Read the model definition and answer for the solid it produces. Units are mm, in the model's axes. Coordinates: 2 decimals unless noted, no trailing zeros. Write each loop counter-clockwise with the first axis right and the second up, starting at its lowest first coordinate (ties: lowest second). Pieces come first, ordered by that corner, then holes.
Item 1: Straight lines are drawn through the part: probe 1 along Z at (x, y) = (-29.75, 6.15); probe 2 along X at (y, z) = (7.3, -115); probe 3 along Z at (x, y) = (-59, 5.95). For each, find the intervals that lie inside material, in ascending order.
Item 2: Each of these flat-tipped pins is pushed along its axis until it touches: P1, Ø1.4, axis at x = -59.75, z = -108, coming from the -Y side; P2, Ø3, axis at x = -29.75, z = -115, coming from the +Y side. Where does it stop, or does it pass through?
Item 3: Section A-A (z = -115) is taken. Give the vertices of the cut face in (x, y), then the cut area to 3 significant figures.
Item 4: Section B-B (x = -59.75) is taken. Give the vertices of the cut face in (y, z).
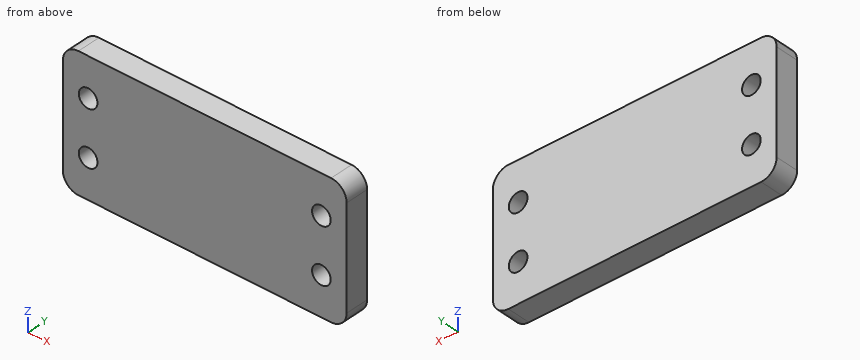
from build123d import *

# Parameters (mm, degrees)
CYLINDER015_R     = 1.2
CYLINDER015_DEPTH = 10
CYLINDER016_R     = 1.2
CYLINDER016_DEPTH = 10
CYLINDER012_R     = 1.2
CYLINDER012_DEPTH = 10
CYLINDER014_R     = 1.2
CYLINDER014_DEPTH = 10
BOX007_W          = 36.5
BOX007_H          = 3
BOX007_DEPTH      = 17
FILLET008_R       = 2


with BuildPart() as m2s002:
    # Cylinder015 → Cylinder015 (new body)
    with BuildSketch(Plane.XZ):
        Circle(CYLINDER015_R)
    extrude(amount=CYLINDER015_DEPTH)


with BuildPart() as fusion018:
    # Cylinder016 → Cylinder016 (new body)
    with BuildSketch(Plane(origin=(30, 0, 0), x_dir=(1, 0, 0), z_dir=(0, -1, 0))):
        Circle(CYLINDER016_R)
    extrude(amount=CYLINDER016_DEPTH)

    # Fusion018: union m2s002
    add(m2s002.part)


with BuildPart() as fusion018_1:
    # Fusion018 placement: moved
    add(fusion018.part.moved(Location((3.25, 0, 7))))


with BuildPart() as m2s:
    # Cylinder012 → Cylinder012 (new body)
    with BuildSketch(Plane.XZ):
        Circle(CYLINDER012_R)
    extrude(amount=CYLINDER012_DEPTH)


with BuildPart() as fusion019:
    # Cylinder014 → Cylinder014 (new body)
    with BuildSketch(Plane(origin=(30, 0, 0), x_dir=(1, 0, 0), z_dir=(0, -1, 0))):
        Circle(CYLINDER014_R)
    extrude(amount=CYLINDER014_DEPTH)

    # Fusion017: union m2s
    add(m2s.part)


with BuildPart() as fusion019_1:
    # Fusion017 placement: moved
    add(fusion019.part.moved(Location((3.25, 0, 0))))

    # Fusion019: union Fusion018
    add(fusion018_1.part)


with BuildPart() as fusion019_2:
    # Fusion019 placement: moved
    add(fusion019_1.part.moved(Location((0, 3, 5))))


with BuildPart() as convertersupport:
    # Box007 → Box007 (new body)
    with BuildSketch(Plane.XY):
        with Locations((18.25, 1.5)):
            Rectangle(BOX007_W, BOX007_H)
    extrude(amount=BOX007_DEPTH)

    # Cut003: cut Fusion019
    add(fusion019_2.part, mode=Mode.SUBTRACT)

    # Fillet008
    fillet008_edges = [convertersupport.edges().sort_by_distance(p)[0] for p in [
        (0, 1.5, 17),
        (0, 1.5, 0),
        (36.5, 1.5, 17),
        (36.5, 1.5, 0),
    ]]
    fillet(fillet008_edges, radius=FILLET008_R)


with BuildPart() as convertersupport_1:
    # Fillet008 placement: moved
    add(convertersupport.part.moved(Location((-63, 5, -120))))


solid = convertersupport_1.part
Established:
1. probe 1: z = -120 to -116.2, -113.8 to -109.2, -106.8 to -103
1. probe 2: x = -63 to -60.95, -58.55 to -30.95, -28.55 to -26.5
1. probe 3: z = -120 to -115.94, -114.06 to -108.94, -107.06 to -103
2. P1: passes through
2. P2: stops at y = 8
3. outline: (-63, 5) - (-60.95, 5) - (-60.95, 8) - (-63, 8) - close; (-58.55, 5) - (-30.95, 5) - (-30.95, 8) - (-58.55, 8) - close; (-28.55, 5) - (-26.5, 5) - (-26.5, 8) - (-28.55, 8) - close
3. area: 95.1 mm2
4. outline: (5, -120) - (8, -120) - (8, -116.2) - (5, -116.2) - close; (5, -113.8) - (8, -113.8) - (8, -109.2) - (5, -109.2) - close; (5, -106.8) - (8, -106.8) - (8, -103) - (5, -103) - close
